Work out the finished part from the listing and answer in its coordinate system (mm). A direction names the side the tool comes from. Round coordinates to 2 decimals unless told otherwise and drop trailing zeros. Loops run counter-clockwise (first coordinate to the right, second up) from the corner with the lowest first, then second, coordinate; pieces in that order, holes last. Notation, with made-up numbers: (10, 72) - (63, 72) arc R17 ccw to (63, 103) - close; hole circle Ø7 at (6.25, 10). An arc over 180 degrees is marked (long way). Answer as CSV lines item,"result". Start each with the question number.
Q1. Each of these flat-tipped pins is pushed along its axis until it touches: pin 1 Ø2.5 at (x, y) = (-23.1, -7) entering from -Z; pin 2 Ø1.8 at (x, z) = (-23.5, 3.5) entering from +Y. Where does it stop, or does it pass through?
Q2. Straight lines are drawn through the part: L1, parallel to Y at x = -23.1, z = 3.9; L2, parallel to Y at x = -22.25, z = 1.5; L3, parallel to Y at x = -17, z = 0.65. For each, find the intervals that lie inside material, in ascending order. Write a range as [from, to].
Q3. Section A-A on z = 5.15 is taken. Write down the section's boundary in (x, y), then the cut area to 3 significant figures.
Q4. Section D-D on y = -0.75 is taken. Write down the section's boundary in (x, z).
Q5. Section C-C on y = -8 is taken. Write down the section's boundary in (x, z).
Q6. Section B-B on x = -17.3 is taken. Write down the section's boundary in (y, z), then the cut area to 3 significant figures.
Q7. The mould has two halves that part along Y. Classify faces 1 (the face through (-17.4, 6.8, 3)), 2 (the face through (-20, -7, 0)), 3 (the face through (-16.053, -17.483, 2.958)), 4 (the face through (-23, -18, 3)): +Y half, -Y half, draft (parallel to the pull), parting line (faces both ways), or undercut.
Q8. For faces 5 (the face through (-23, 4, 3)), 6 (the face through (-14.5, -7, 3)), determine the directions among +Z, -Z, +X, -X, +Y, -Y from which every point of the face is accessible in a straight line to the end or side of a thin tool.
Autodesk Inventor part; units mm, degrees
ref_plane "YZ Plane" through (0, 0, 0) normal (1, 0, 0) x (0, 1, 0)
ref_plane "XZ Plane" through (0, 0, 0) normal (0, 1, 0) x (-1, 0, 0)
ref_plane "XY Plane" through (0, 0, 0) normal (0, 0, 1) x (1, 0, 0)
ref_plane "작업 평면1" through (0, 0, 0) normal (0, 0, 1) x (1, 0, 0)
sketch "스케치1" plane through (0, 0, 0) normal (0, 0, 1) x (1, 0, 0)
  line L0 (-15, 14.5) -> (-11.5, 14.5)
  line L1 (-15, 14.5) -> (-20.1, 8.5)
  line L2 (-20.1, 8.5) -> (-20.1, -44.6)
  line L3 (-20.1, -44.6) -> (-15, -50.6)
  line L4 (-15, -50.6) -> (15, -50.6)
  line L5 (15, -50.6) -> (20.1, -44.6)
  line L6 (20.1, -44.6) -> (20.1, 8.5)
  line L7 (20.1, 8.5) -> (15, 14.5)
  line L8 (11.5, 14.5) -> (15, 14.5)
  arc A0 (14.5, 11.5) -> (11.5, 14.5) centre (11.5, 11.5) ccw
  line L9 (14.5, -42) -> (14.5, 11.5)
  arc A1 (11.5, -45) -> (14.5, -42) centre (11.5, -42) ccw
  line L10 (-11.5, -45) -> (11.5, -45)
  arc A2 (-14.5, -42) -> (-11.5, -45) centre (-11.5, -42) ccw
  line L11 (-14.5, 11.5) -> (-14.5, -42)
  arc A3 (-11.5, 14.5) -> (-14.5, 11.5) centre (-11.5, 11.5) ccw
  circle A4 centre (17.3, 4) radius 1.35
  circle A5 centre (17.3, -18) radius 1.35
  circle A6 centre (17.3, -40) radius 1.35
  circle A7 centre (11, -47.8) radius 1.35
  circle A8 centre (-17.3, 4) radius 1.35
  circle A9 centre (-17.3, -18) radius 1.35
  circle A10 centre (-17.3, -40) radius 1.35
  circle A11 centre (-11, -47.8) radius 1.35
  circle A12 centre (-17.3, -18) radius 2.8
  circle A13 centre (-17.3, 4) radius 2.8
  line L12 (-20.1, -18) -> (-20.1, 4)
  line L13 (-20.1, 4) -> (-26.1, 4)
  line L14 (-26.1, 4) -> (-26.1, -18)
  line L15 (-26.1, -18) -> (-20.1, -18)
  line L16 (-26.1, -18) -> (-26.1, -7)
  line L17 (-23.1, -18) -> (-23.1, -12.5)
  line L18 (-23.1, 4) -> (-23.1, -1.5)
  line L19 (-23.1, -1.5) -> (-23.1, -7)
  circle A14 centre (-23.1, -12.5) radius 1.35
  circle A15 centre (-23.1, -7) radius 1.35
  circle A16 centre (-23.1, -1.5) radius 1.35
  point P0 (0, 0)
  point P1 (-14.5, -18)
  point P2 (-14.5, 4)
  dimension "d0" = 6
  dimension "d1" = 11
  dimension "d2" = 5.5
  dimension "d3" = 2.7
  dimension "d4" = 2.7
  dimension "d5" = 2.7
extrude "돌출1" add sketch "스케치1" along normal blind 6 contours A13 L11 A12 L2 | A13 | L2 L15 L14 L13 | A12
properties part number "_idle_adt"
Findings:
1,pin 1,"passes through"
1,pin 2,"stops at y = 4"
2,L1,"y = [-18, -13.85], [-11.15, -8.35], [-5.65, -2.85], [-0.15, 4]"
2,L2,"y = [-18, -13.55], [-11.45, -8.05], [-5.95, -2.55], [-0.45, 4]"
2,L3,"y = [-20.78, -19.32], [-16.68, 2.68], [5.32, 6.78]"
3,outline,"(-26.1, -18) - (-20.1, -18) arc R2.8 ccw to (-14.5, -18) - (-14.5, 4) arc R2.8 ccw to (-20.1, 4) - (-26.1, 4) - close; hole circle Ø2.7 at (-23.1, -12.5); hole circle Ø2.7 at (-23.1, -7); hole circle Ø2.7 at (-23.1, -1.5); hole circle Ø2.7 at (-17.3, -18); hole circle Ø2.7 at (-17.3, 4)"
3,area,"251 mm^2"
4,outline,"(-26.1, 0) - (-24.22, 0) - (-24.22, 6) - (-26.1, 6) - close; (-21.98, 0) - (-14.5, 0) - (-14.5, 6) - (-21.98, 6) - close"
5,outline,"(-26.1, 0) - (-24.01, 0) - (-24.01, 6) - (-26.1, 6) - close; (-22.19, 0) - (-14.5, 0) - (-14.5, 6) - (-22.19, 6) - close"
6,outline,"(-20.8, 0) - (-19.35, 0) - (-19.35, 6) - (-20.8, 6) - close; (-16.65, 0) - (2.65, 0) - (2.65, 6) - (-16.65, 6) - close; (5.35, 0) - (6.8, 0) - (6.8, 6) - (5.35, 6) - close"
6,area,"133 mm^2"
7,face 1,"+Y half"
7,face 2,"draft"
7,face 3,"undercut"
7,face 4,"-Y half"
8,face 5,"+Z, -Z, -X, +Y"
8,face 6,"+Z, -Z, +X, +Y, -Y"
